Read the model definition and answer for the solid it produces. Units are mm, in the model's axes. A direction names the side the tool comes from. Coordinates: 2 decimals unless noted, no trailing zeros. Write each loop counter-clockwise with the first axis right and the second up, starting at its lowest first coordinate (ties: lowest second). Pieces come first, ordered by that corner, then holes.
(1) Section A-A on x = -1.25 is taken. Write down the section's boundary in (y, z).
(2) Which of the six approach directions +Z, -Z, +X, -X, +Y, -Y give full straight-line access (tool end or side, diameter ignored) to faces 5 (the flat face through (4.5, 0, 0)), 6 (the flat face through (0, 0, -0.25))?
(3) Section B-B on y = 1.75 is taken. Write down the section's boundary in (x, z), then the cut area to 3 significant figures.
(4) Find the intervals of material crossed by probe 1 along Z at (x, y) = (3.75, -10.75); probe 2 along X at (y, z) = (-13.25, -0.65), in increasing order.
(5) The mould has two halves that part along Z. Classify faces 1 (the flat face through (0, 0, 1.25)), 2 (the flat face through (-4.5, 0, 0)), 3 (the flat face through (0, 0, 0.75)), 4 (the flat face through (0, 0, -1.25)): +Z half, -Z half, draft (parallel to the pull), parting line (faces both ways), or undercut.
from build123d import *

# Parameters (mm, degrees)
SKETCH1_W           = 9
SKETCH1_H           = 2.5
BOSS_EXTRUDE1_DEPTH = 15
CUT_EXTRUDE1_START  = -31
SKETCH2_W           = 8
SKETCH2_H           = 0.5
CUT_EXTRUDE1_DEPTH  = 32


with BuildPart() as part:
    # Sketch1 → Boss-Extrude1 (new body, symmetric)
    with BuildSketch(Plane(origin=(0, 0, 0), x_dir=(1, 0, 0), z_dir=(0, 1, 0))):
        Rectangle(SKETCH1_W, SKETCH1_H)
    extrude(amount=BOSS_EXTRUDE1_DEPTH, both=True)

    # Sketch2 → Cut-Extrude1 (cut)
    with BuildSketch(Plane(origin=(0, 15, 0), x_dir=(1, 0, 0), z_dir=(0, 1, 0)).offset(CUT_EXTRUDE1_START)):
        with Locations((0, 0.5)):
            Rectangle(SKETCH2_W, SKETCH2_H)
    cut_extrude1 = extrude(amount=CUT_EXTRUDE1_DEPTH, mode=Mode.SUBTRACT)

    # Mirror1: Cut-Extrude1 across plane
    add(cut_extrude1.mirror(Plane.XY), mode=Mode.SUBTRACT)


solid = part.part
Response:
1. outline: (-15, -1.25) - (15, -1.25) - (15, -0.75) - (-15, -0.75) - close; (-15, -0.25) - (15, -0.25) - (15, 0.25) - (-15, 0.25) - close; (-15, 0.75) - (15, 0.75) - (15, 1.25) - (-15, 1.25) - close
2. face 5: +Z, -Z, +X, +Y, -Y
2. face 6: +Y, -Y
3. outline: (-4.5, -1.25) - (4.5, -1.25) - (4.5, 1.25) - (-4.5, 1.25) - close; hole (-4, -0.75) - (4, -0.75) - (4, -0.25) - (-4, -0.25) - close; hole (-4, 0.25) - (4, 0.25) - (4, 0.75) - (-4, 0.75) - close
3. area: 14.5 mm2
4. probe 1: z = -1.25 to -0.75, -0.25 to 0.25, 0.75 to 1.25
4. probe 2: x = -4.5 to -4, 4 to 4.5
5. face 1: +Z half
5. face 2: draft
5. face 3: undercut
5. face 4: -Z half
